CAD build for the part. Positions are in the model's coordinates, mm. Round coordinates to 2 decimals unless told otherwise and drop trailing zeros. Loops run counter-clockwise (first coordinate to the right, second up) from the corner with the lowest first, then second, coordinate; pieces in that order, holes last.
from build123d import *

# Parameters (mm, degrees)
F0_W     = 115
F0_H     = 70
F1_DEPTH = 6
F3_D     = 15
F3_DEPTH = 20
F4_D     = 5.8
F4_DEPTH = 20
F5_D     = 6
F5_DEPTH = 20
F6_SIZE  = 0.5


with BuildPart() as f1:
    # F0 (on Top) → F1 (new body)
    with BuildSketch(Plane.XY):
        Rectangle(F0_W, F0_H)
    extrude(amount=F1_DEPTH)

    # F3
    with Locations(Plane.XY.offset(6)):
        with Locations((-43.5, -3)):
            Hole(F3_D / 2, depth=F3_DEPTH)

    # F4
    with Locations(Plane.XY.offset(6)):
        with Locations((-43.5, 25), (-43.5, -25)):
            Hole(F4_D / 2, depth=F4_DEPTH)

    # F5
    with Locations(Plane.XY.offset(6)):
        with Locations((40, 20), (40, -20)):
            Hole(F5_D / 2, depth=F5_DEPTH)

    # F6
    f6_edges = [f1.edges().sort_by_distance(p)[0] for p in [
        (0, -35, 0),
        (-57.5, 0, 0),
        (57.5, 0, 0),
        (0, 35, 0),
        (-46.4, -25, 0),
        (-51, -3, 0),
        (37, -20, 0),
        (-46.4, 25, 0),
        (37, 20, 0),
        (0, -35, 6),
        (-57.5, 0, 6),
        (57.5, 0, 6),
        (0, 35, 6),
        (-46.4, -25, 6),
        (-51, -3, 6),
        (37, -20, 6),
        (-46.4, 25, 6),
        (37, 20, 6),
        (57.5, 35, 3),
        (57.5, -35, 3),
        (-57.5, -35, 3),
        (-57.5, 35, 3),
    ]]
    chamfer(f6_edges, length=F6_SIZE)


solid = f1.part
Item 1: Cut at A-A (y = -25). List the corners of the cut face in (x, z).
Verdict:
outline: (-57.5, 0.5) - (-57, 0) - (-46.9, 0) - (-46.4, 0.5) - (-46.4, 5.5) - (-46.9, 6) - (-57, 6) - (-57.5, 5.5) - close; (-40.6, 0.5) - (-40.1, 0) - (57, 0) - (57.5, 0.5) - (57.5, 5.5) - (57, 6) - (-40.1, 6) - (-40.6, 5.5) - close
Item 2: Cut at C-C (z = 4.25). List the corners of the cut face in (x, y), plus the area to 3 significant figures.
Verdict:
outline: (-57.5, -34.5) - (-57, -35) - (57, -35) - (57.5, -34.5) - (57.5, 34.5) - (57, 35) - (-57, 35) - (-57.5, 34.5) - close; hole circle Ø15 at (-43.5, -3); hole circle Ø5.8 at (-43.5, -25); hole circle Ø5.8 at (-43.5, 25); hole circle Ø6 at (40, -20); hole circle Ø6 at (40, 20)
area: 7,760 mm2
Item 3: Mould opens along Y. For faces 1 (the flat face through (-1, -35, 3)), 2 (the flat face through (57.5, 0, 3)), 3 (the cylindrical face through (43, -20, 3)), 4 (the cylindrical face through (-46.18, 23.89, 2.96)) say: released by +Y, released by -Y, zero draft, split by the parting line, or undercut.
Verdict:
face 1: released by -Y
face 2: zero draft
face 3: undercut
face 4: undercut
Item 4: Wall check: L1, parallel to Y at x = -43.5, z = 2.2; L2, parallel to Y at x = 40, z = 1.6; L3, parallel to X at y = -27, z = 5.75. Give the ranges that are in metal, low to high.
Verdict:
L1: y = -35 to -27.9, -22.1 to -10.5, 4.5 to 22.1, 27.9 to 35
L2: y = -35 to -23, -17 to 17, 23 to 35
L3: x = -57.25 to -45.93, -41.07 to 57.25
Item 5: Cut at B-B (x = -43.5). State how many separate pieces and enclosed holes the cut face has, plus the area to 3 significant figures.
Verdict:
separate pieces: 4
enclosed holes: 0
area: 258 mm2
Item 6: Cut at D-D (x = 40). List the corners of the cut face in (y, z).
Verdict:
outline: (-35, 0.5) - (-34.5, 0) - (-23.5, 0) - (-23, 0.5) - (-23, 5.5) - (-23.5, 6) - (-34.5, 6) - (-35, 5.5) - close; (-17, 0.5) - (-16.5, 0) - (16.5, 0) - (17, 0.5) - (17, 5.5) - (16.5, 6) - (-16.5, 6) - (-17, 5.5) - close; (23, 0.5) - (23.5, 0) - (34.5, 0) - (35, 0.5) - (35, 5.5) - (34.5, 6) - (23.5, 6) - (23, 5.5) - close
